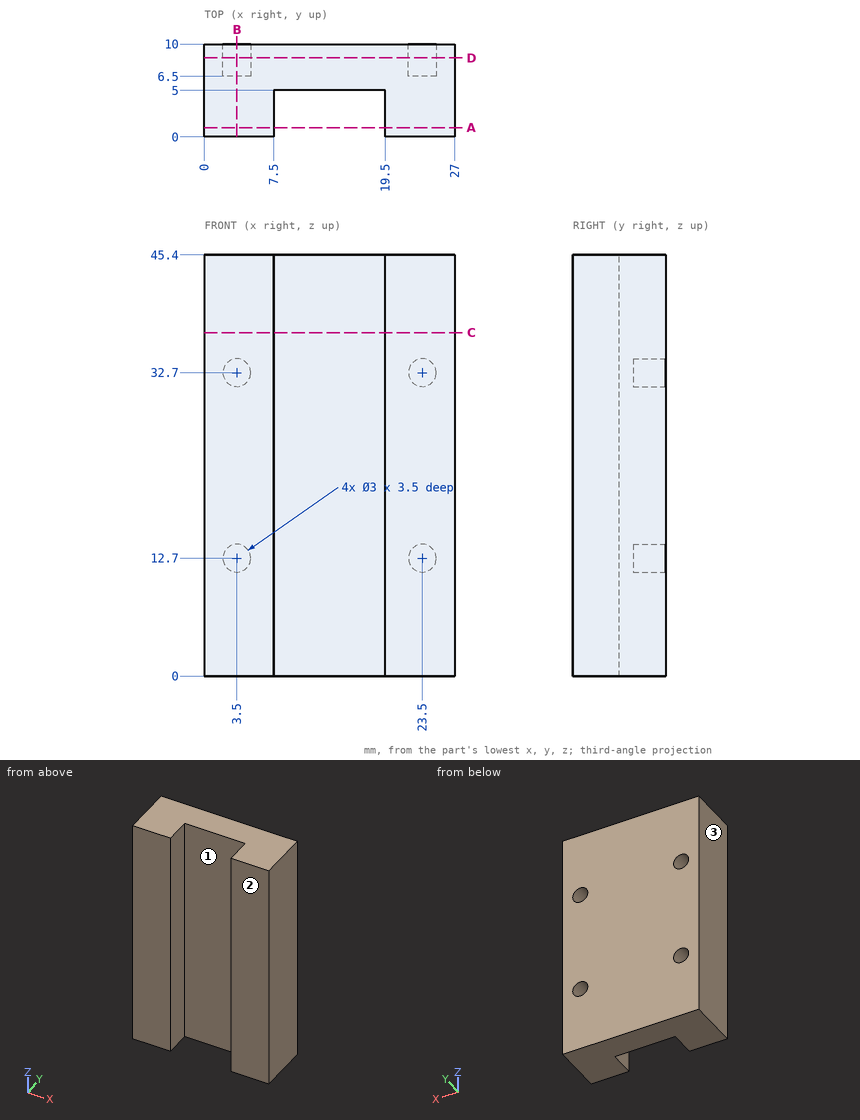
Input: dimensioned drawing with shaded views. Units: mm. Origin: part minimum x, y, z. Round coordinates to 2 decimals unless told otherwise and drop trailing zeros. Loops run counter-clockwise (first coordinate to the right, second up) from the corner with the lowest first, then second, coordinate; pieces in that order, holes last. Notation, with made-up numbers: M -10.5,-13.75 L 20.5,-13.75 A22 ccw 20.5,18.25 Z; hole C -28.5,-21 d8. An arc over 180 degrees is marked long. Return JSON: item names as keys, results as strings. Group by question number.
1. Material intervals for line 1 along Z through (x, y) = (23.5, 8.1); line 2 along X through (y, z) = (8.85, 32.7); line 3 along X through (y, z) = (4.25, 42.5), sorted ascending. Write a range as from..to.
2. Section query A-A on y = 1. Output: boundary loops of the cut face in (x, z), and give its area (3 significant figures).
3. Pin query (flat end, axial travel): pin 1 (1.5 mm diameter, centred on x = 12.5, z = 22.5, fed in from -Y); pin 2 (2.5 mm diameter, centred on x = 23.5, z = 32.7, fed in from +Y). Return the tip coordinate at first contact, or that it passes through.
4. Mould query, pull axis X, two halves, no side actions, for the marked faces 1, 2 and 3. Classes: released by +X, released by -X, zero draft, split by the parting line, or undercut.
5. Section query C-C on z = 37. Output: boundary loops of the cut face in (x, y), and give its area (3 significant figures).
6. Section query B-B on x = 3.5. Output: boundary loops of the cut face in (y, z).
7. Section query D-D on y = 8.5. Output: boundary loops of the cut face in (x, z).
Checks:
{
 "1": {"line 1": "z = 0..11.2, 14.2..31.2, 34.2..45.4", "line 2": "x = 0..2, 5..22, 25..27", "line 3": "x = 0..7.5, 19.5..27"},
 "2": {"outline": "M 0,0 L 7.5,0 L 7.5,45.4 L 0,45.4 Z; M 19.5,0 L 27,0 L 27,45.4 L 19.5,45.4 Z", "area": "681 mm²"},
 "3": {"pin 1": "stops at y = 5", "pin 2": "stops at y = 6.5"},
 "4": {"face 1": "undercut", "face 2": "zero draft", "face 3": "released by -X"},
 "5": {"outline": "M 0,0 L 7.5,0 L 7.5,5 L 19.5,5 L 19.5,0 L 27,0 L 27,10 L 0,10 Z", "area": "210 mm²"},
 "6": {"outline": "M 0,0 L 10,0 L 10,11.2 L 6.5,11.2 L 6.5,14.2 L 10,14.2 L 10,31.2 L 6.5,31.2 L 6.5,34.2 L 10,34.2 L 10,45.4 L 0,45.4 Z"},
 "7": {"outline": "M 0,0 L 27,0 L 27,45.4 L 0,45.4 Z; hole C 3.5,12.7 d3; hole C 3.5,32.7 d3; hole C 23.5,12.7 d3; hole C 23.5,32.7 d3"}
}
